Design review of the part built by this model. Coordinates are the model's own, in mm. Coordinates: 2 decimals unless noted, no trailing zeros. Loops run counter-clockwise (first coordinate to the right, second up) from the corner with the lowest first, then second, coordinate; pieces in that order, holes last. Notation, with made-up numbers: (72, 80) -> (120, 80) arc R17 ccw to (120, 85) -> close; hole circle Ø11 at (27.25, 56). An arc over 180 degrees is marked (long way). One line per item, written item: value. Start each with the question number.
1. Add section C-C on x = 12. Write out the cut boundary in (y, z), plus the area to 3 significant figures.
2. Insertion check: pin 1 (1.8 mm diameter, centred on x = 71, z = 9, fed in from -Y). The pin has a flat end and moves straight along its axis. Give the tip position at first contact, or say it passes through.
3. Draft analysis for pull direction X (two halves, no side actions). For faces 1 (the flat face through (39, 1, 0)), 2 (the cylindrical face through (69.614, 1.479, 9.575)), 3 (the flat face through (80, 1, 13)), state which applies: pulls with the +X half, pulls with the -X half, needs draft (parallel to the pull), parting line crosses it, or undercut.
4. Add section A-A on x = 71. Write out the cut boundary in (y, z), plus the area to 3 significant figures.
5. Add section B-B on y = 0.7. Write out the cut boundary in (x, z).
6. For probe 1 along X at (y, z) = (1.9, 9); probe 2 along Z at (x, y) = (26, 0.6); probe 3 along X at (y, z) = (1.7, 9.5), list the stretches that pass through material, from the lowest coordinate up.
```python
from build123d import *

# Parameters (mm, degrees)
SKETCH1_W                   = 80
SKETCH1_H                   = 25
BOSS_EXTRUDE1_DEPTH         = 3
F_3_0MM_PRESS_DOWEL_HOLE1_D = 3
F_5_0MM_PRESS_DOWEL_HOLE1_D = 5


with BuildPart() as part:
    # Sketch1 → Boss-Extrude1 (new body)
    with BuildSketch(Plane(origin=(0, 0, 0), x_dir=(1, 0, 0), z_dir=(0, 1, 0))):
        with Locations((40, -12.5)):
            Rectangle(SKETCH1_W, SKETCH1_H)
    extrude(amount=BOSS_EXTRUDE1_DEPTH)

    # Ø3.0mm Press Dowel Hole1 (through all)
    with Locations(Plane(origin=(0, 3, 0), x_dir=(1, 0, 0), z_dir=(0, 1, 0))):
        with Locations((71, -9), (56, -9), (41, -9), (26, -9)):
            Hole(F_3_0MM_PRESS_DOWEL_HOLE1_D / 2)

    # Ø5.0mm Press Dowel Hole1 (through all)
    with Locations(Plane(origin=(0, 3, 0), x_dir=(1, 0, 0), z_dir=(0, 1, 0))):
        with Locations((12, -9)):
            Hole(F_5_0MM_PRESS_DOWEL_HOLE1_D / 2)


solid = part.part
```
Worked answers:
1. outline: (0, 0) -> (3, 0) -> (3, 6.5) -> (0, 6.5) -> close; (0, 11.5) -> (3, 11.5) -> (3, 25) -> (0, 25) -> close
1. area: 60.0 mm²
2. pin 1: passes through
3. face 1: needs draft
3. face 2: undercut
3. face 3: pulls with the +X half
4. outline: (0, 0) -> (3, 0) -> (3, 7.5) -> (0, 7.5) -> close; (0, 10.5) -> (3, 10.5) -> (3, 25) -> (0, 25) -> close
4. area: 66.0 mm²
5. outline: (0, 0) -> (80, 0) -> (80, 25) -> (0, 25) -> close; hole circle Ø5 at (12, 9); hole circle Ø3 at (26, 9); hole circle Ø3 at (41, 9); hole circle Ø3 at (56, 9); hole circle Ø3 at (71, 9)
6. probe 1: x = 0 to 9.5, 14.5 to 24.5, 27.5 to 39.5, 42.5 to 54.5, 57.5 to 69.5, 72.5 to 80
6. probe 2: z = 0 to 7.5, 10.5 to 25
6. probe 3: x = 0 to 9.55, 14.45 to 24.59, 27.41 to 39.59, 42.41 to 54.59, 57.41 to 69.59, 72.41 to 80
